Could you check a few things on this drawing? It's one solid part, dimensions in mm from its lowest x, y, z. Round coordinates to 2 decimals unless told otherwise and drop trailing zeros. Write each loop counter-clockwise with the first axis right and the second up, starting at its lowest first coordinate (ties: lowest second). Pieces come first, ordered by that corner, then holes. Notation, with made-up numbers: M 88.5,52.5 L 138.5,52.5 A18 cw 138.5,77.5 Z; hole C 48.5,3.5 d4. An arc over 180 degrees is marked long. One line per question, with ' | ' between items. Start each with the question number.
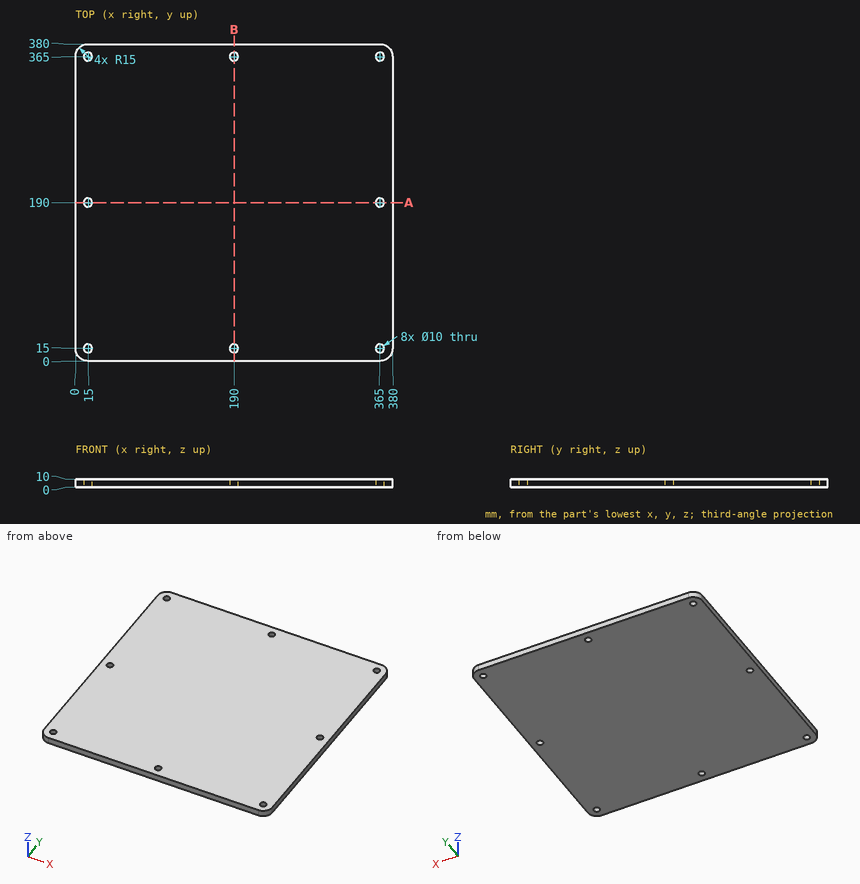
1. I need wall thicknesses on line 1 along Y through (x, z) = (190, 5.75); line 2 along X through (y, z) = (365, 8). Which ranges of each line are inside material? Lowest first, please. Write a range as from..to.
2. Suppose I cut it at A-A (y = 190). Write out the boundary of the cut face in (x, z), and give its area (3 significant figures).
Computed:
1) line 1: y = 0..10, 20..360, 370..380 | line 2: x = 0..10, 20..185, 195..360, 370..380
2) outline: M 0,0 L 10,0 L 10,10 L 0,10 Z; M 20,0 L 360,0 L 360,10 L 20,10 Z; M 370,0 L 380,0 L 380,10 L 370,10 Z | area: 3,600 mm²
